Can you work these out from the model? Positions are in its coordinate system, mm. A direction names the side the tool comes from. Give positions to 0.01 mm unless a question says otherwise; leave off trailing zeros. Loops run counter-clockwise (first coordinate to the right, second up) from the corner with the lowest first, then second, coordinate; pieces in that order, holes last. Notation, with made-up numbers: (7, 39.25) -> (25, 39.25) arc R34 cw to (25, 75.25) -> close; hole circle Ø5 at (37.25, 76.5). An arc over 180 degrees is marked (long way). One line per question, with ' | ' between items.
from build123d import *

# Parameters (mm, degrees)
SKETCH_1_W          = 100
SKETCH_1_H          = 15
EXTRUDE_1_DEPTH     = 15
SHELL_1_T           = -3.01271481
EXTRUDE_2_DEPTH     = 3
SKETCH_4_R          = 2.15
CUT_EXTRUDE_1_DEPTH = 4.01271481
EXTRUDE_3_DEPTH     = 3
SKETCH_6_R          = 2.15
CUT_EXTRUDE_2_DEPTH = 4.01271481


with BuildPart() as part:
    # 草图1 → 凸台-拉伸1 (new body)
    with BuildSketch(Plane(origin=(0, 0, 0), x_dir=(1, 0, 0), z_dir=(0, 1, 0))):
        with Locations((50, 7.5)):
            Rectangle(SKETCH_1_W, SKETCH_1_H)
    extrude(amount=EXTRUDE_1_DEPTH)

    # 抽壳1
    shell_1_openings = [part.faces().sort_by_distance(p)[0] for p in [
        (50, 15, -7.5),
    ]]
    offset(amount=SHELL_1_T, openings=shell_1_openings, kind=Kind.INTERSECTION)

    # 草图3 → 凸台-拉伸2 (add)
    with BuildSketch(Plane(origin=(3.01271481, 0, 0), x_dir=(0, 0, -1), z_dir=(1, 0, 0))):
        Polygon((1.85, 4.713912937), (7.5, 1.451883916), (13.15, 4.713912937), (13.15, 11.237970979), (7.5, 14.5), (1.85, 11.237970979), align=None)
        Polygon((7.5, 3.761284993), (11.15, 5.868613476), (11.15, 10.083270441), (7.5, 12.190598923), (3.85, 10.083270441), (3.85, 5.868613476), align=None, mode=Mode.SUBTRACT)
    extrude(amount=EXTRUDE_2_DEPTH)

    # 草图4 → 切除-拉伸1 (cut, through all)
    with BuildSketch(Plane(origin=(3.01271481, 0, 0), x_dir=(0, 0, -1), z_dir=(1, 0, 0))):
        with Locations((7.5, 7.975941958)):
            Circle(SKETCH_4_R)
    extrude(amount=-CUT_EXTRUDE_1_DEPTH, mode=Mode.SUBTRACT)

    # 草图5 → 凸台-拉伸3 (add)
    with BuildSketch(Plane.ZY.offset(-96.98728519)):
        Polygon((-3.01271481, 11.909264688), (-7.5, 14.5), (-11.98728519, 11.909264688), (-11.98728519, 4.042619229), (-10.20343841, 3.01271481), (-4.79656159, 3.01271481), (-3.01271481, 4.042619229), align=None)
        Polygon((-11.15, 10.083270441), (-7.5, 12.190598923), (-3.85, 10.083270441), (-3.85, 5.868613476), (-7.5, 3.761284993), (-11.15, 5.868613476), align=None, mode=Mode.SUBTRACT)
    extrude(amount=EXTRUDE_3_DEPTH)

    # 草图6 → 切除-拉伸2 (cut, through all)
    with BuildSketch(Plane.ZY.offset(-96.98728519)):
        with Locations((-7.5, 7.975941958)):
            Circle(SKETCH_6_R)
    extrude(amount=-CUT_EXTRUDE_2_DEPTH, mode=Mode.SUBTRACT)


solid = part.part
Q1. For pin 1 Ø2.5 at (y, z) = (7.98, -7.5) entering from -X; pin 2 Ø2.5 at (x, z) = (47, -6) entering from +Y, each with a flat end and sliding along its axis, tell me the tip position at first contact or that it passes through.
Entries:
pin 1: through | pin 2: y = 3.01
Q2. On a 3-axis mill with a long thin cutter (end or side, diameter ignored), from which of +Z, -Z, +X, -X, +Y, -Y can I reach the whole of each face in a straight line? I mean faces 5 (the face through (6.013, 11.4, -9.4)), 6 (the face through (49, 15, -13)), 7 (the face through (4.49, 3.52, -11.08)). Say none if no direction works.
Entries:
face 5: +Y | face 6: +Z, -Z, +X, -X, +Y | face 7: none
Q3. If we section it at A-A (z = -6.5): Write out the boundary of the cut face in (x, y).
Entries:
outline: (0, 0) -> (100, 0) -> (100, 6.07) -> (96.99, 6.07) -> (96.99, 4.34) -> (93.99, 4.34) -> (93.99, 3.01) -> (6.01, 3.01) -> (6.01, 4.34) -> (3.01, 4.34) -> (3.01, 6.07) -> (0, 6.07) -> close; (0, 9.88) -> (3.01, 9.88) -> (3.01, 11.61) -> (6.01, 11.61) -> (6.01, 13.92) -> (3.01, 13.92) -> (3.01, 15) -> (0, 15) -> close; (93.99, 11.61) -> (96.99, 11.61) -> (96.99, 9.88) -> (100, 9.88) -> (100, 15) -> (96.99, 15) -> (96.99, 13.92) -> (93.99, 13.92) -> close
Q4. If I drill on probe 1 along Z at (x, y) = (17.5, 5.5); probe 2 along Y at (x, z) = (98.7, -7.5); probe 3 along X at (y, z) = (4, -9.75), over which ranges is the centre line in solid material (lowest first)? Write a range as from..to.
Entries:
probe 1: -15..-11.99, -3.01..0 | probe 2: 0..5.83, 10.13..15 | probe 3: 0..6.01, 93.99..100
Q5. If we section it at B-B (x = 74): Write out the boundary of the cut face in (y, z), plus the area to 3 significant figures.
Entries:
outline: (0, -15) -> (15, -15) -> (15, -11.99) -> (3.01, -11.99) -> (3.01, -3.01) -> (15, -3.01) -> (15, 0) -> (0, 0) -> close | area: 117 mm²
Q6. If we mould it in two halves opening along X, with no side actions, what happens to faces 1 (the face through (95.51, 11.15, -5.7)), 2 (the face through (100, 6, -6)), 3 (the face through (49, 7, 0)), 4 (the face through (0, 6, -6))? For each: pulls with the +X half, pulls with the -X half, needs draft (parallel to the pull), parting line crosses it, or undercut.
Entries:
face 1: undercut | face 2: pulls with the +X half | face 3: needs draft | face 4: pulls with the -X half
